from build123d import *

# Parameters (mm, degrees)
SKETCH1_W                       = 38.1
SKETCH1_H                       = 38.1
BOSS_EXTRUDE1_DEPTH             = 12.7
SKETCH2_R                       = 7.62
CUT_EXTRUDE1_DEPTH              = 0.127
TAP_DRILL_FOR_1_4_20_TAP2_D     = 5.1054
TAP_DRILL_FOR_1_4_20_TAP2_DEPTH = 6.35
TAP_DRILL_FOR_1_4_20_TAP2_TIP   = 1.533816902


with BuildPart() as part:
    # Sketch1 → Boss-Extrude1 (new body)
    with BuildSketch(Plane(origin=(0, 0, 0), x_dir=(1, 0, 0), z_dir=(0, 1, 0))):
        Rectangle(SKETCH1_W, SKETCH1_H)
    extrude(amount=BOSS_EXTRUDE1_DEPTH)

    # Sketch2 → Cut-Extrude1 (cut)
    with BuildSketch(Plane(origin=(0, 12.7, 0), x_dir=(1, 0, 0), z_dir=(0, 1, 0))):
        with Locations(Location((0, 0, 0), (0, 0, 270))):
            Circle(SKETCH2_R)
    extrude(amount=-CUT_EXTRUDE1_DEPTH, mode=Mode.SUBTRACT)

    # Tap Drill for 1/4-20 Tap2
    with Locations(Plane(origin=(0, 12.7, 0), x_dir=(1, 0, 0), z_dir=(0, 1, 0))):
        with Locations((-13.97, 13.97), (13.97, 13.97), (13.97, -13.97), (-13.97, -13.97)):
            Hole(TAP_DRILL_FOR_1_4_20_TAP2_D / 2, depth=TAP_DRILL_FOR_1_4_20_TAP2_DEPTH)
            with Locations((0, 0, -(TAP_DRILL_FOR_1_4_20_TAP2_DEPTH + TAP_DRILL_FOR_1_4_20_TAP2_TIP / 2))):  # 118° drill point
                Cone(0, TAP_DRILL_FOR_1_4_20_TAP2_D / 2, TAP_DRILL_FOR_1_4_20_TAP2_TIP, mode=Mode.SUBTRACT)


solid = part.part
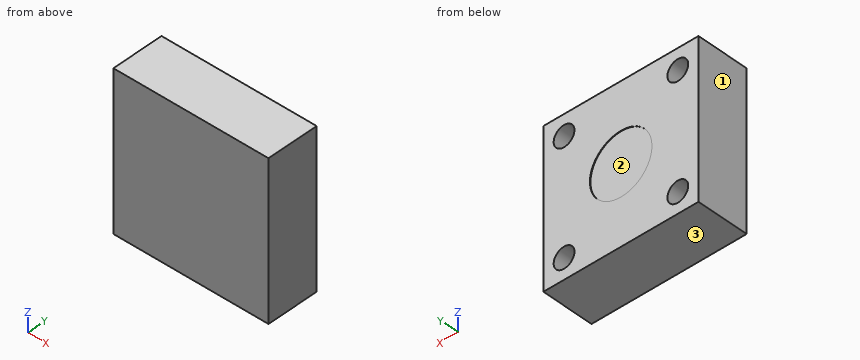
For this review, take the finished solid that the model builds, in its own axes (mm). Face numbers are marked on the shaded views. Round coordinates to 2 decimals unless told otherwise and drop trailing zeros. Loops run counter-clockwise (first coordinate to the right, second up) from the corner with the lowest first, then second, coordinate; pieces in that order, holes last. Notation, with made-up numbers: (33, 58.5) - (73, 58.5) arc R20 ccw to (73, 69.5) - close; hole circle Ø7 at (23, 20). An arc over 180 degrees is marked (long way). One line per item, written item: value. Start each with the question number.
Item 1: For L1, parallel to X at y = 11, z = -13.97; L2, parallel to X at y = 7, z = -16, list the stretches that pass through material, from the lowest coordinate up.
Item 2: Take a section at A-A (y = 8). Give the boundary of the cut face in (x, z), plus the area to 3 significant figures.
Item 3: The part is to be moulded in two halves that separate along X. For the marked faces 1, 2 and 3, say which applies: +X half, -X half, draft (parallel to the pull), parting line (faces both ways), or undercut.
Item 4: Take a section at B-B (y = 5.75). Give the boundary of the cut face in (x, z), plus the area to 3 significant figures.
Answer below:
1. L1: x = -19.05 to -16.52, -11.42 to 11.42, 16.52 to 19.05
1. L2: x = -19.05 to -15.52, -12.42 to 12.42, 15.52 to 19.05
2. outline: (-19.05, -19.05) - (19.05, -19.05) - (19.05, 19.05) - (-19.05, 19.05) - close; hole circle Ø5.11 at (-13.97, -13.97); hole circle Ø5.11 at (-13.97, 13.97); hole circle Ø5.11 at (13.97, -13.97); hole circle Ø5.11 at (13.97, 13.97)
2. area: 1,370 mm2
3. face 1: -X half
3. face 2: undercut
3. face 3: draft
4. outline: (-19.05, -19.05) - (19.05, -19.05) - (19.05, 19.05) - (-19.05, 19.05) - close; hole circle Ø3.11 at (-13.97, -13.97); hole circle Ø3.11 at (-13.97, 13.97); hole circle Ø3.11 at (13.97, -13.97); hole circle Ø3.11 at (13.97, 13.97)
4. area: 1,420 mm2
